```python
from build123d import *

# Parameters (mm, degrees)
SKETCH_1_W          = 71.5
SKETCH_1_H          = 60.5
SKETCH_1_W_2        = 63.5
SKETCH_1_H_2        = 58.5
EXTRUDE_1_DEPTH     = 7
FILLET_1_R          = 2
SKETCH_2_W          = 3
SKETCH_2_H          = 8
CUT_EXTRUDE_1_DEPTH = 7
SKETCH_3_W          = 8
SKETCH_3_H          = 2.5
CUT_EXTRUDE_2_DEPTH = 92.002747211


with BuildPart() as part:
    # Эскиз1 → Бобышка-Вытянуть1 (new body)
    with BuildSketch(Plane(origin=(0, 0, 0), x_dir=(1, 0, 0), z_dir=(0, 1, 0))):
        with Locations((31.75, -29.25)):
            Rectangle(SKETCH_1_W, SKETCH_1_H)
        with Locations((31.75, -29.25)):
            Rectangle(SKETCH_1_W_2, SKETCH_1_H_2, mode=Mode.SUBTRACT)
    extrude(amount=EXTRUDE_1_DEPTH)

    # Скругление1
    fillet_1_edges = [part.edges().sort_by_distance(p)[0] for p in [
        (0, 3.5, 0),
        (0, 3.5, 58.5),
        (63.5, 3.5, 58.5),
        (63.5, 3.5, 0),
    ]]
    fillet(fillet_1_edges, radius=FILLET_1_R)

    # Эскиз2 → Вырез-Вытянуть1 (cut)
    with BuildSketch(Plane(origin=(0, 7, 0), x_dir=(1, 0, 0), z_dir=(0, 1, 0))):
        with Locations((-2.5, -28)):
            Rectangle(SKETCH_2_W, SKETCH_2_H)
        with Locations((66, -28)):
            Rectangle(SKETCH_2_W, SKETCH_2_H)
    extrude(amount=-CUT_EXTRUDE_1_DEPTH, mode=Mode.SUBTRACT)

    # Эскиз3 → Вырез-Вытянуть2 (cut, through all)
    with BuildSketch(Plane(origin=(64.5, 0, 0), x_dir=(0, 0, -1), z_dir=(1, 0, 0))):
        with Locations((-28, 1.25)):
            Rectangle(SKETCH_3_W, SKETCH_3_H)
    extrude(amount=-CUT_EXTRUDE_2_DEPTH, mode=Mode.SUBTRACT)


solid = part.part
```
Geometry check sheet. Reference: the model listing, model coordinates, mm. A direction names the side the tool comes from. Round coordinates to 2 decimals unless told otherwise and drop trailing zeros. Loops run counter-clockwise (first coordinate to the right, second up) from the corner with the lowest first, then second, coordinate; pieces in that order, holes last. Notation, with made-up numbers: (69.5, -25) -> (127.5, -25) arc R20 cw to (127.5, -15) -> close; hole circle Ø4 at (34.25, 75). An arc over 180 degrees is marked (long way). Use a Markdown table: item, result.
(1) Go/stop test with flat-tipped pins: P1, Ø1.3, axis at y = 6, z = 27.5, coming from the -X side; P2, Ø0.5, axis at x = -0.5, z = 27.5, coming from the -Y side; P3, Ø1.3, axis at y = 4, z = 26.5, coming from the +X side; P4, Ø3, axis at y = 2, z = 24.5, coming from the +X side. Record where each tip stops, or that it passes through.
Calculated:
| item | result |
|---|---|
| P1 | x = -1 |
| P2 | y = 2.5 |
| P3 | x = 64.5 |
| P4 | x = 67.5 |
(2) Sectioned sample at A-A (z = 40). Enter the section's corners in (x, y).
Calculated:
| item | result |
|---|---|
| outline | (-4, 0) -> (0, 0) -> (0, 7) -> (-4, 7) -> close; (63.5, 0) -> (67.5, 0) -> (67.5, 7) -> (63.5, 7) -> close |
(3) Set-up check for faces 4 (the flat face through (67.5, 3, 46)), 5 (the cylindrical face through (0.6, 3.55, 0.57)), 6 (the flat face through (64.5, 5, 28)), 7 (the flat face through (31, 3, -1)), 8 (the flat face through (-1, 5, 28)): record each of +Z, -Z, +X, -X, +Y, -Y from which the full face is reachable in a straight line by a thin tool's end or side.
Calculated:
| item | result |
|---|---|
| face 4 | +Z, -Z, +X, +Y, -Y |
| face 5 | +Y, -Y |
| face 6 | +X, +Y, -Y |
| face 7 | -Z, +X, -X, +Y, -Y |
| face 8 | -X, +Y, -Y |
(4) Scan lines: probe 1 along Z at (x, y) = (61, 3.5); probe 2 along X at (y, z) = (1.25, 32.5); probe 3 along X at (y, z) = (4.5, 26.5). Record each from-to range of solid material in increasing order.
Calculated:
| item | result |
|---|---|
| probe 1 | -1 to 0, 58.5 to 59.5 |
| probe 2 | -4 to 0, 63.5 to 67.5 |
| probe 3 | -1 to 0, 63.5 to 64.5 |
(5) Sectioned sample at C-C (y = 5.5). Enter the section's corners in (x, z), then the cut area to 3 significant figures.
Calculated:
| item | result |
|---|---|
| outline | (-4, -1) -> (67.5, -1) -> (67.5, 24) -> (64.5, 24) -> (64.5, 32) -> (67.5, 32) -> (67.5, 59.5) -> (-4, 59.5) -> (-4, 32) -> (-1, 32) -> (-1, 24) -> (-4, 24) -> close; hole (0, 2) arc R2 ccw to (2, 0) -> (61.5, 0) arc R2 ccw to (63.5, 2) -> (63.5, 56.5) arc R2 ccw to (61.5, 58.5) -> (2, 58.5) arc R2 ccw to (0, 56.5) -> close |
| area | 566 mm² |
(6) Sectioned sample at B-B (x = 27). Enter the section's corners in (y, z).
Calculated:
| item | result |
|---|---|
| outline | (0, -1) -> (7, -1) -> (7, 0) -> (0, 0) -> close; (0, 58.5) -> (7, 58.5) -> (7, 59.5) -> (0, 59.5) -> close |
(7) Mould release check, pull along Z, two halves, no side actions. Record for faces 1 (the flat face through (-4, 3, 46)), 2 (the flat face through (31, 3, 59.5)), 3 (the flat face through (-2, 4, 32)): released by +Z, released by -Z, zero draft, split by the parting line, or undercut.
Calculated:
| item | result |
|---|---|
| face 1 | zero draft |
| face 2 | released by +Z |
| face 3 | undercut |
